```python
from build123d import *

# Parameters (mm, degrees)
CORTE_EXTRUS_O1_DEPTH = 1.5


with BuildPart() as part:
    # Esboço1 → Revolução1 (revolve)
    with BuildSketch(Plane(origin=(0, 0, 0), x_dir=(1, 0, 0), z_dir=(0, 1, 0))):
        Polygon((0, 0), (2.75, 0), (2.75, -3), (1.5, -3), (1.5, -9), (0, -9), (0, -3), align=None)
    revolve(axis=Axis((0, 0, 3), (0, 0, -1)))

    # Esboço2 → Corte-extrusão1 (cut)
    with BuildSketch(Plane(origin=(0, 0, 0), x_dir=(-1, 0, 0), z_dir=(0, 0, -1))):
        Polygon((1.732050808, 0), (0.866025404, 1.5), (-0.866025404, 1.5), (-1.732050808, 0), (-0.866025404, -1.5), (0.866025404, -1.5), align=None)
    extrude(amount=-CORTE_EXTRUS_O1_DEPTH, mode=Mode.SUBTRACT)


solid = part.part
```
CAD build for the part. Positions are in the model's coordinates, mm. A direction names the side the tool comes from. Give positions to 0.01 mm unless a question says otherwise; leave off trailing zeros. Order: outer loops, then holes, each group sorted by start corner. A loop starts at its lowest first (then second) coordinate and runs counter-clockwise, first axis right, second up.
(1) Saw through at D-D, the plane z = 5.25. Give the cut face in (x, y).
(2) Saw through at C-C, the plane z = 1.75. Give the cut face in (x, y), then the cut area to 3 significant figures.
(3) Saw through at B-B, the plane y = -1.35. Give the cut face in (x, z), then the cut area to 3 significant figures.
(4) Tool access for faces 1 (the flat face through (-1.293, -0.76, 0.74)), 2 (the cylindrical face through (-1.5, -0.07, 6.04)), 3 (the flat face through (-2, 0, 0)): list every direction of +Z, -Z, +X, -X, +Y, -Y with a clear straight run to the whole face (end or side of a thin tool).
(5) Flat gauge pins, fed straight in: pin 1 (1 mm diameter, centred on y = -0.5, z = 4.5, fed in from +X); pin 2 (0.9 mm diameter, centred on x = 0, y = -0.5, fed in from -Z); pin 3 (3 mm diameter, centred on x = 1, z = 6.5, fed in from -Y). Where does each tip first touch, or does it go through?
(6) Drill centre lines: L1, parallel to Z at x = -0.8, y = 2.4; L2, parallel to Z at x = 0.35, y = 1.15; L3, parallel to X at y = -1.25, z = 0.5. Where is each one in solid material? Low to high.
(7) Mould opens along X. For faces 4 (the flat face through (1.305, -0.74, 0.74)), 5 (the flat face through (1.2, 1.2, 3)), 6 (the cylindrical face through (-0.596, 2.685, 1.521)) say: released by +X, released by -X, zero draft, split by the parting line, or undercut.
(8) Saw through at A-A, the plane x = 0. Give the cut face in (y, z).
Results found:
1. outline: circle Ø3 at (0, 0)
2. outline: circle Ø5.5 at (0, 0)
2. area: 23.8 mm2
3. outline: (-2.4, 0) - (-0.95, 0) - (-0.95, 1.5) - (0.95, 1.5) - (0.95, 0) - (2.4, 0) - (2.4, 3) - (0.65, 3) - (0.65, 9) - (-0.65, 9) - (-0.65, 3) - (-2.4, 3) - close
3. area: 19.4 mm2
4. face 1: -Z
4. face 2: +Z
4. face 3: -Z, +X, -X, +Y, -Y
5. pin 1: stops at x = 1.5
5. pin 2: stops at z = 1.5
5. pin 3: stops at y = -1.5
6. L1: z = 0 to 3
6. L2: z = 1.5 to 9
6. L3: x = -2.45 to -1.01, 1.01 to 2.45
7. face 4: undercut
7. face 5: zero draft
7. face 6: split by the parting line
8. outline: (-2.75, 0) - (-1.5, 0) - (-1.5, 1.5) - (1.5, 1.5) - (1.5, 0) - (2.75, 0) - (2.75, 3) - (1.5, 3) - (1.5, 9) - (-1.5, 9) - (-1.5, 3) - (-2.75, 3) - close
